Could you check a few things on this model? Use its own coordinates, in mm. Face numbers are marked on the shaded views. A direction names the side the tool comes from. Give positions to 0.01 mm unless a question says otherwise; leave off trailing zeros. Order: outer loops, then holes, each group sorted by start corner. A loop starts at its lowest first (then second) coordinate and runs counter-clockwise, first axis right, second up. Notation, with made-up numbers: (15.5, 82.5) -> (73.5, 82.5) arc R19 ccw to (73.5, 118.5) -> close; hole circle Ø5 at (81.5, -34). An arc over 180 degrees is marked (long way). Use one line per item in the form item = value. Start each with the question number.
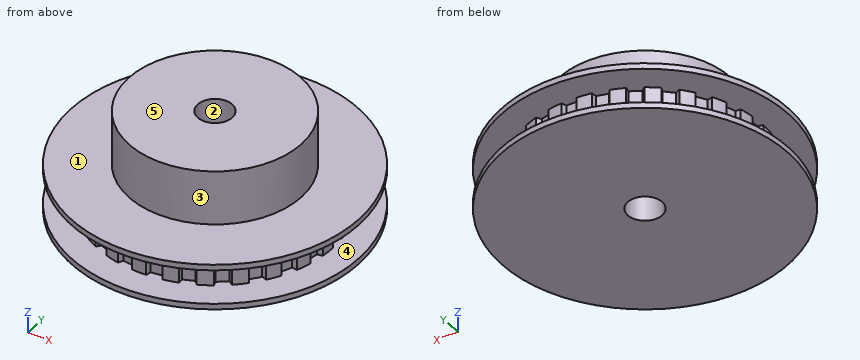
from build123d import *

# Parameters (mm, degrees)
SKETCH2_R           = 20.417784581
BOSS_EXTRUDE1_DEPTH = 3
CUT_EXTRUDE3_DEPTH  = 6
SKETCH5_R           = 25
BOSS_EXTRUDE2_DEPTH = 1
SKETCH6_R           = 15
BOSS_EXTRUDE3_DEPTH = 9.5
SKETCH8_R           = 3
CUT_EXTRUDE4_DEPTH  = 40.449334595


with BuildPart() as part:
    # Sketch2 → Boss-Extrude1 (new, symmetric)
    with BuildSketch(Plane.XY):
        Circle(SKETCH2_R)
    extrude(amount=BOSS_EXTRUDE1_DEPTH, both=True)

    # Sketch4 → Cut-Extrude3 (cut)
    with BuildSketch(Plane.XY.offset(3)):
        Polygon((1.006646689, 19.511049769), (1.376859102, 20.528200014), (-1.376813629, 20.528075077), (-1.006601216, 19.510924833), align=None)
        Polygon((5.827221798, 18.647731411), (6.438758286, 19.540857927), (3.771566178, 20.225547476), (3.877192707, 19.148284794), align=None)
        Polygon((10.28165113, 16.612707507), (11.096086608, 17.32569187), (8.682964611, 18.652174343), (8.517368354, 17.582487599), align=None)
        Polygon((14.090046509, 13.533846092), (15.056206999, 14.021888874), (13.048780443, 15.906816498), (12.622366422, 14.911918045), align=None)
        Polygon((17.013112445, 9.604603354), (18.070290531, 9.837039031), (16.59469341, 12.161974871), (15.934254785, 11.304377837), align=None)
        Polygon((18.867181957, 5.071868063), (19.948951252, 5.034091847), (19.09790076, 7.652951634), (18.244935319, 6.986541995), align=None)
        Polygon((19.535757038, 0.22044865), (20.574145998, -0.085165841), (20.401116767, 2.663065301), (19.409219466, 2.229716025), align=None)
        Polygon((18.976828657, -4.644822364), (19.906591485, -5.199072246), (20.422455578, -2.49415122), (19.353950973, -2.667211203), align=None)
        Polygon((17.225516339, -9.218242105), (17.988232618, -9.986301822), (19.160576396, -7.494651046), (18.08260256, -7.396547742), align=None)
        Polygon((14.391861479, -13.212445793), (14.939606939, -14.146055326), (16.694767732, -12.024234384), (15.675057726, -11.661131984), align=None)
        Polygon((10.653913032, -16.37646292), (10.952270812, -17.416960149), (13.179965412, -15.798290853), (12.282591366, -15.193004416), align=None)
        Polygon((6.246540048, -18.511486653), (6.27676323, -19.593493311), (8.837017393, -18.579682606), (8.118364618, -17.770244505), align=None)
        Polygon((1.446673978, -19.483365599), (1.20686353, -20.538895228), (3.93880707, -20.19364457), (3.444031164, -19.230914778), align=None)
        Polygon((-3.444091937, -19.23103303), (-3.938867844, -20.193762822), (-1.206892986, -20.538765578), (-1.446703434, -19.483235948), align=None)
        Polygon((-8.11845289, -17.770343928), (-8.837105665, -18.579782029), (-6.276759518, -19.593360409), (-6.246536335, -18.51135375), align=None)
        Polygon((-12.28270159, -15.193078763), (-13.180075636, -15.7983652), (-10.952234165, -17.416832345), (-10.653876385, -16.376335116), align=None)
        Polygon((-15.675182977, -11.661176583), (-16.694892983, -12.024278984), (-14.939539659, -14.145940651), (-14.391794199, -13.212331118), align=None)
        Polygon((-18.082734968, -7.396559792), (-19.160708804, -7.494663096), (-17.988138933, -9.986207481), (-17.225422655, -9.218147765), align=None)
        Polygon((-19.354082217, -2.667189946), (-20.422586822, -2.494129963), (-19.906477283, -5.199004168), (-18.976714454, -4.644754285), align=None)
        Polygon((-19.409341301, 2.229769254), (-20.401238602, 2.663118529), (-20.574018453, -0.085128303), (-19.535629493, 0.220486188), align=None)
        Polygon((-18.245040089, 6.98662385), (-19.098005529, 7.653033489), (-19.948818379, 5.034096487), (-18.867049084, 5.071872703), align=None)
        Polygon((-15.934335907, 11.304483176), (-16.594774532, 12.162080209), (-18.070160678, 9.837010481), (-17.012982592, 9.604574804), align=None)
        Polygon((-12.622418798, 14.912040248), (-13.04883282, 15.906938701), (-15.056088326, 14.021828928), (-14.089927835, 13.533786146), align=None)
        Polygon((-8.517388694, 17.582618989), (-8.682984951, 18.652305732), (-11.095986571, 17.325604294), (-10.281551093, 16.612619931), align=None)
        Polygon((-3.877179733, 19.148417114), (-3.771553204, 20.225679796), (-6.438683171, 19.540748224), (-5.827146683, 18.647621709), align=None)
    extrude(amount=-CUT_EXTRUDE3_DEPTH, mode=Mode.SUBTRACT)

    # Sketch5 → Boss-Extrude2 (add)
    with BuildSketch(Plane.XY.offset(3)):
        Circle(SKETCH5_R)
    boss_extrude2 = extrude(amount=BOSS_EXTRUDE2_DEPTH)

    # Mirror2: Boss-Extrude2 across plane
    add(boss_extrude2.mirror(Plane.XY))

    # Sketch6 → Boss-Extrude3 (add)
    with BuildSketch(Plane.XY.offset(4)):
        Circle(SKETCH6_R)
    extrude(amount=BOSS_EXTRUDE3_DEPTH)

    # Sketch8 → Cut-Extrude4 (cut, through all)
    with BuildSketch(Plane.XY.offset(13.5)):
        Circle(SKETCH8_R)
    extrude(amount=-CUT_EXTRUDE4_DEPTH, mode=Mode.SUBTRACT)


solid = part.part
(1) Imagine slicing it at B-B (z = 12.25). Write out the boundary of the cut face in (x, y).
(2) I'm going to push flat-ended pins straight in: pin 1 Ø3 at (x, z) = (-18, 6.5) entering from -Y; pin 2 Ø2 at (y, z) = (-9.5, 7.5) entering from -X; pin 3 Ø5 at (y, z) = (0, 10.5) entering from -X; pin 4 Ø9.5 at (x, y) = (0, 0) entering from -Z. Where does each tip first touch, or does it pass through?
(3) Imagine slicing it at A-A (x = 0). Write out the boundary of the cut face in (y, z), plus the area to 3 significant figures.
(4) Please list where these lines run through material, in increasing order: probe 1 along Y at (x, z) = (0, 9.75); probe 2 along Y at (x, z) = (0, 2); probe 3 along Z at (x, y) = (17.5, -3).
(5) We'd pull the mould along Y, two halves only. Please class the marked faces 1, 2 and 3: pulls with the +Y half, pulls with the -Y half, needs draft (parallel to the pull), parting line crosses it, or undercut.
(6) Which directions (+Z, -Z, +X, -X, +Y, -Y) give clear straight access to the entire face, cutting with the end or side of a thin tool? Please do the marked faces 4 and 5.
(7) Imagine slicing it at C-C (x = 9.5). Write out the boundary of the cut face in (y, z), plus the area to 3 significant figures.
(8) Imagine slicing it at D-D (x = 21.5). Write out the boundary of the cut face in (y, z).
Calculated:
q1.outline = circle Ø30 at (0, 0); hole circle Ø6 at (0, 0)
q2.pin_1 = through
q2.pin_2 = -12.36
q2.pin_3 = -15
q2.pin_4 = -4
q3.outline = (-25, -4) -> (-3, -4) -> (-3, 13.5) -> (-15, 13.5) -> (-15, 4) -> (-25, 4) -> (-25, 3) -> (-20.42, 3) -> (-20.42, -3) -> (-25, -3) -> close; (3, -4) -> (25, -4) -> (25, -3) -> (19.51, -3) -> (19.51, 3) -> (25, 3) -> (25, 4) -> (15, 4) -> (15, 13.5) -> (3, 13.5) -> close
q3.area = 520 mm2
q4.probe_1 = -15 to -3, 3 to 15
q4.probe_2 = -20.42 to -3, 3 to 19.51
q4.probe_3 = -4 to 4
q5.face_1 = needs draft
q5.face_2 = undercut
q5.face_3 = parting line crosses it
q6.face_4 = none
q6.face_5 = +Z, +X, -X, +Y, -Y
q7.outline = (-23.12, -4) -> (23.12, -4) -> (23.12, -3) -> (17.04, -3) -> (17.04, 3) -> (23.12, 3) -> (23.12, 4) -> (11.61, 4) -> (11.61, 13.5) -> (-11.61, 13.5) -> (-11.61, 4) -> (-23.12, 4) -> (-23.12, 3) -> (-18.07, 3) -> (-18.07, -3) -> (-23.12, -3) -> close
q7.area = 524 mm2
q8.outline = (-12.76, -4) -> (12.76, -4) -> (12.76, -3) -> (-12.76, -3) -> close; (-12.76, 3) -> (12.76, 3) -> (12.76, 4) -> (-12.76, 4) -> close
